Input: part model. Units: mm. Frame: model coordinates. Coordinates: 2 decimals unless noted, no trailing zeros. Loops run counter-clockwise (first coordinate to the right, second up) from the corner with the lowest first, then second, coordinate; pieces in that order, holes last. Notation, with made-up numbers: (80, -12.5) - (124, -12.5) arc R3 cw to (124, -8.5) - close; hole circle Ø10 at (-9.5, -13.75). An arc over 180 degrees is marked (long way). Use a Markdown table: item, result. Add a question column.
1. Contact query for flat-ended pins moving along their axis: P1, Ø3, axis at x = 126.5, z = 114.5, coming from the -Y side; P2, Ø4, axis at x = -41.5, z = 143.5, coming from the +Y side; P3, Ø8, axis at x = -12.5, z = 80.5, coming from the +Y side. Output: stop coordinate, or through.
2. Ray query, L1, parallel to X at y = -51, z = 79.5; L2, parallel to Z at x = 101.5, y = 94.5; L3, parallel to X at y = -34.5, z = 39.5. Return the intervals inside material, ascending. Write a range as [from, to].
3. Section query A-A on z = 262. Return the cut outline in (x, y).
```python
from build123d import *

# Parameters (mm, degrees)
F0_R     = 225
F1_DEPTH = 500
F5_SCALE = 0.75


with BuildPart() as f1:
    # F0 (on Top) → F1 (new body)
    with BuildSketch(Plane.XY):
        Circle(F0_R)
    extrude(amount=F1_DEPTH)

    # F2 (on Front) → F4 (revolve, cut)
    with BuildSketch(Plane.XZ):
        with BuildLine():
            Line((-370.3630566597, 0), (-87.1822908521, 0))
            add(Edge.make_bspline(
                [(-87.1822908521, 0), (-90.6749721594, 3.8222254673), (-94.0881927527, 7.6209101654), (-97.4234330683, 11.3993561694)],
                knots=[0, 0, 0, 0, 13.9758277665, 13.9758277665, 13.9758277665, 13.9758277665], degree=3))
            add(Edge.make_bspline(
                [(-97.4234330683, 11.3993561694), (-220.0127632021, 150.279053206), (-237.2517737021, 261.8165432768), (-222.6538360119, 509.9815130234)],
                knots=[13.9758277665, 13.9758277665, 13.9758277665, 13.9758277665, 527.6681563005, 527.6681563005, 527.6681563005, 527.6681563005], degree=3))
            Line((-222.6538360119, 509.9815130234), (-370.3630566597, 526.1934995651))
            Line((-370.3630566597, 526.1934995651), (-370.3630566597, 0))
        make_face()
        with BuildLine():
            add(Edge.make_bspline(
                [(-87.1822908521, 0), (-90.6749721594, 3.8222254673), (-94.0881927527, 7.6209101654), (-97.4234330683, 11.3993561694)],
                knots=[0, 0, 0, 0, 13.9758277665, 13.9758277665, 13.9758277665, 13.9758277665], degree=3))
            Line((-87.1822908521, 0), (-97.4234330683, 11.3993561694))
        make_face()
    revolve(axis=Axis((0, 0, 313.555), (0, 0, 1)), mode=Mode.SUBTRACT)


with BuildPart() as f1_1:
    # F5: moved
    add(f1.part.scale(F5_SCALE))


solid = f1_1.part
```
Resolved:
| question | item | result |
|---|---|---|
| 1 | P1 | y = -68.62 |
| 1 | P2 | y = 148 |
| 1 | P3 | y = 127.36 |
| 2 | L1 | [-114.26, 114.26] |
| 2 | L2 | [105.87, 375] |
| 2 | L3 | [-92.24, 92.24] |
| 3 | outline | circle Ø337.5 at (0, 0) |
